from build123d import *

# Parameters (mm, degrees)
CROQUIS1_W                         = 44.45
CROQUIS1_H                         = 63.5
BRIDA_BASE1_DEPTH                  = 1.524
BRIDA_DE_ARISTA1_STRIP_W           = 9.144
BRIDA_DE_ARISTA1_STRIP_H           = 1.524
BRIDA_DE_ARISTA1_STRIP_CUT_DEPTH   = 63.5
BRIDA_DE_ARISTA1_STRIP_2_W         = 9.144
BRIDA_DE_ARISTA1_STRIP_2_H         = 1.524
BRIDA_DE_ARISTA1_STRIP_CUT_2_DEPTH = 63.5
BRIDA_DE_ARISTA1_DEPTH             = 63.5
BRIDA_DE_ARISTA1_BEND_DEPTH        = 63.5
CROQUIS12_R                        = 3.175
CROQUIS12_W                        = 16.002
CROQUIS12_H                        = 25.4
CORTAR_EXTRUIR1_DEPTH              = 62.738
CROQUIS13_R                        = 3.5687
CORTAR_EXTRUIR2_DEPTH              = 62.738
CORTAR_EXTRUIR3_DEPTH              = 62.738


# Sheet-metal steps are written as plain solids
with BuildPart() as part:
    # Croquis1 → Brida base1 (new body)
    with BuildSketch(Plane.XY):
        Rectangle(CROQUIS1_W, CROQUIS1_H)
    extrude(amount=-BRIDA_BASE1_DEPTH)

    # Brida de arista1 strip (across the edge) → Brida de arista1 strip cut (cut)
    with BuildSketch(Plane(origin=(22.225, -31.75, 0), x_dir=(-1, 0, 0), z_dir=(0, 1, 0))):
        with Locations((-1.524, -0.762)):
            Rectangle(BRIDA_DE_ARISTA1_STRIP_W, BRIDA_DE_ARISTA1_STRIP_H)
    extrude(amount=BRIDA_DE_ARISTA1_STRIP_CUT_DEPTH, mode=Mode.SUBTRACT)

    # Brida de arista1 strip 2 (across the edge) → Brida de arista1 strip cut 2 (cut)
    with BuildSketch(Plane(origin=(-22.225, 31.75, 0), x_dir=(1, 0, 0), z_dir=(0, -1, 0))):
        with Locations((-1.524, -0.762)):
            Rectangle(BRIDA_DE_ARISTA1_STRIP_2_W, BRIDA_DE_ARISTA1_STRIP_2_H)
    extrude(amount=BRIDA_DE_ARISTA1_STRIP_CUT_2_DEPTH, mode=Mode.SUBTRACT)

    # Brida de arista1 section (across the edge) → Brida de arista1 (add)
    with BuildSketch(Plane(origin=(22.225, -31.75, 0), x_dir=(-1, 0, 0), z_dir=(0, 1, 0))):
        with BuildLine():
            Line((0, 1.524), (0, 27.178))
            Line((0, 27.178), (1.524, 27.178))
            Line((1.524, 27.178), (1.524, 1.524))
            ThreePointArc((1.524, 1.524), (1.970369265, 0.446369265), (3.048, 0))
            Line((3.048, 0), (3.048, -1.524))
            ThreePointArc((3.048, -1.524), (0.892738531, -0.631261469), (0, 1.524))
        make_face()
    extrude(amount=BRIDA_DE_ARISTA1_DEPTH)

    # Brida de arista1 section 2 (across the edge) → Brida de arista1 bend (add)
    with BuildSketch(Plane(origin=(-22.225, 31.75, 0), x_dir=(1, 0, 0), z_dir=(0, -1, 0))):
        with BuildLine():
            Line((0, 1.524), (0, 27.178))
            Line((0, 27.178), (1.524, 27.178))
            Line((1.524, 27.178), (1.524, 1.524))
            ThreePointArc((1.524, 1.524), (1.970369265, 0.446369265), (3.048, 0))
            Line((3.048, 0), (3.048, -1.524))
            ThreePointArc((3.048, -1.524), (0.892738531, -0.631261469), (0, 1.524))
        make_face()
    extrude(amount=BRIDA_DE_ARISTA1_BEND_DEPTH)

    # Croquis12 → Cortar-Extruir1 (cut)
    with BuildSketch(Plane(origin=(22.225, 0, 0), x_dir=(0, 0, -1), z_dir=(1, 0, 0))):
        with Locations((-20.828, 22.352)):
            Circle(CROQUIS12_R)
        with Locations((-6.477, 19.05)):
            Rectangle(CROQUIS12_W, CROQUIS12_H)
    extrude(amount=-CORTAR_EXTRUIR1_DEPTH, mode=Mode.SUBTRACT)

    # Croquis13 → Cortar-Extruir2 (cut)
    with BuildSketch(Plane(origin=(0, 0, -1.524), x_dir=(-1, 0, 0), z_dir=(0, 0, -1))):
        with Locations((0, -22.098)):
            Circle(CROQUIS13_R)
        with Locations((0, -3.048)):
            Circle(CROQUIS13_R)
    extrude(amount=-CORTAR_EXTRUIR2_DEPTH, mode=Mode.SUBTRACT)

    # Croquis14 → Cortar-Extruir3 (cut)
    with BuildSketch(Plane(origin=(22.225, 0, 0), x_dir=(0, 0, -1), z_dir=(1, 0, 0))):
        Polygon((-14.478, 31.75), (-16.986914912, 31.75), (-14.478, 29.241085088), align=None)
        Polygon((-27.178, 31.75), (-24.669085088, 31.75), (-27.178, 29.241085088), align=None)
    extrude(amount=-CORTAR_EXTRUIR3_DEPTH, mode=Mode.SUBTRACT)


solid = part.part
Source: CAD feature listing. Evaluate the final solid. Frame: model axes, mm. A direction names the side the tool comes from. Coordinates: 2 decimals unless noted, no trailing zeros. Loops run counter-clockwise (first coordinate to the right, second up) from the corner with the lowest first, then second, coordinate; pieces in that order, holes last. Notation, with made-up numbers: (8.25, 44) -> (38.25, 44) arc R24 cw to (38.25, 71) -> close; hole circle Ø9 at (12, 63). An arc over 180 degrees is marked (long way). Answer in a Markdown table with one row per item. Add a question column.
Q1. Section A-A on y = 15. Return the cut outline in (x, z) (3 decimals).
Q2. Reachability of faces 1 (the face through (0, 6.35, -1)), 2 (the face through (21, -2, 27.178)), 3 (the face through (20.27, -12.97, 0.46)) from +Z, -Z, +X, -X, +Y, -Y: full face, straight path, thin tool, end or side. Return the list, or none.
Q3. Section C-C on z = 0.75. Return the cut outline in (x, y), and give its area (3 significant figures).
Q4. Section B-B on x = 0. Return the cut outline in (y, z), and give its area (3 significant figures).
Q5. Ray query, line 1 along Y through (x, z) = (0, -1.05); line 2 along X through (y, z) = (18, 23.25) (3 decimals); line 3 along Z through (x, y) = (-5, 4.5). Return the intervals inside material, ascending.
Q6. Contact query for flat-ended pins moving along their axis: pin 1 Ø6.5 at (x, y) = (0, -3.048) entering from +Z; pin 2 Ø7.5 at (y, z) = (22.352, 20.828) entering from -X (3 decimals); pin 3 Ø0.8 at (x, y) = (21.5, 12) entering from -Z. Output: stop coordinate, or through.
Q7. Pull-direction query (X, two-part tool) for faces 4 (the face through (21.47, 25.5, 21.24)), 5 (the face through (21.308, -12.967, -0.655)), 6 (the face through (0, -12, 0)); classes: pulls with the +X half, pulls with the -X half, needs draft (parallel to the pull), parting line crosses it, or undercut.
Q8. Section D-D on y = -10. Return the cut outline in (x, z) (3 decimals).
Computed values:
| question | item | result |
|---|---|---|
| 1 | outline | (-22.225, 14.478) -> (-20.701, 14.478) -> (-20.701, 27.178) -> (-22.225, 27.178) -> close; (20.701, 14.478) -> (22.225, 14.478) -> (22.225, 27.178) -> (20.701, 27.178) -> close |
| 2 | face 1 | -Z, +X, -X, +Y |
| 2 | face 2 | +Z, +X, -X, +Y, -Y |
| 2 | face 3 | +Z, +Y, -Y |
| 3 | outline | (-22.13, -31.75) -> (-20.49, -31.75) -> (-20.49, 6.35) -> (-22.13, 6.35) -> close; (20.49, -31.75) -> (22.13, -31.75) -> (22.13, 6.35) -> (20.49, 6.35) -> close |
| 3 | area | 125 mm^2 |
| 4 | outline | (-31.75, -1.52) -> (-25.67, -1.52) -> (-25.67, 0) -> (-31.75, 0) -> close; (-18.53, -1.52) -> (-6.62, -1.52) -> (-6.62, 0) -> (-18.53, 0) -> close; (0.52, -1.52) -> (6.35, -1.52) -> (6.35, 0) -> (0.52, 0) -> close |
| 4 | area | 36.3 mm^2 |
| 5 | line 1 | y = -31.75 to -25.67, -18.53 to -6.62, 0.52 to 6.35 |
| 5 | line 2 | x = -22.225 to -20.701, 20.701 to 22.225 |
| 5 | line 3 | z = -1.52 to 0 |
| 6 | pin 1 | passes through |
| 6 | pin 2 | stops at x = -22.225 |
| 6 | pin 3 | stops at z = 14.48 |
| 7 | face 4 | needs draft |
| 7 | face 5 | pulls with the +X half |
| 7 | face 6 | undercut |
| 8 | outline | (-22.225, 1.524) arc R3.048 ccw to (-19.177, -1.524) -> (19.177, -1.524) arc R3.048 ccw to (22.225, 1.524) -> (22.225, 27.178) -> (20.701, 27.178) -> (20.701, 1.524) arc R1.524 cw to (19.177, 0) -> (-19.177, 0) arc R1.524 cw to (-20.701, 1.524) -> (-20.701, 27.178) -> (-22.225, 27.178) -> close |
